For this review, take the finished solid that the model builds, in its own axes (mm). A direction names the side the tool comes from. Coordinates: 2 decimals unless noted, no trailing zeros. Write each loop counter-clockwise with the first axis right and the second up, starting at its lowest first coordinate (ties: lowest second). Pieces come first, ordered by that corner, then holes.
```python
from build123d import *

# Parameters (mm, degrees)
F0_W     = 19.05
F0_H     = 19.05
F1_DEPTH = 5.08
F2_W     = 16.51
F2_H     = 16.51
F3_DEPTH = 20.32
F5_DEPTH = 25.4
F6_SIZE  = 2.54
F7_SIZE  = 1.27


with BuildPart() as f1:
    # F0 (on Top) → F1 (new body)
    with BuildSketch(Plane.XY):
        with Locations((9.525, 9.525)):
            Rectangle(F0_W, F0_H)
    extrude(amount=F1_DEPTH)

    # F2 (on face) → F3 (join)
    with BuildSketch(Plane.XY.offset(5.08)):
        with Locations((9.525, 9.525)):
            Rectangle(F2_W, F2_H)
    extrude(amount=F3_DEPTH)

    # F4 (on face) → F5 (cut)
    with BuildSketch(Plane.XY.offset(25.4)):
        with BuildLine():
            Line((5.0348719395, 5.0348719395), (9.525, 9.525))
            Line((9.525, 9.525), (5.0348719395, 14.0151280605))
            ThreePointArc((5.0348719395, 14.0151280605), (3.175, 9.525), (5.0348719395, 5.0348719395))
        make_face()
        with BuildLine():
            Line((5.0348719395, 14.0151280605), (9.525, 9.525))
            Line((9.525, 9.525), (14.0151280605, 14.0151280605))
            ThreePointArc((14.0151280605, 14.0151280605), (9.525, 15.875), (5.0348719395, 14.0151280605))
        make_face()
        with BuildLine():
            Line((9.525, 9.525), (14.0151280605, 5.0348719395))
            ThreePointArc((14.0151280605, 5.0348719395), (15.3916350314, 7.0949602045), (15.875, 9.525))
            ThreePointArc((15.875, 9.525), (15.3916350314, 11.9550397955), (14.0151280605, 14.0151280605))
            Line((14.0151280605, 14.0151280605), (9.525, 9.525))
        make_face()
        with BuildLine():
            ThreePointArc((5.0348719395, 5.0348719395), (9.525, 3.175), (14.0151280605, 5.0348719395))
            Line((14.0151280605, 5.0348719395), (9.525, 9.525))
            Line((9.525, 9.525), (5.0348719395, 5.0348719395))
        make_face()
    extrude(amount=-F5_DEPTH, mode=Mode.SUBTRACT)

    # F6
    f6_edges = [f1.edges().sort_by_distance(p)[0] for p in [
        (17.78, 17.78, 15.24),
        (1.27, 17.78, 15.24),
        (1.27, 1.27, 15.24),
        (17.78, 1.27, 15.24),
    ]]
    chamfer(f6_edges, length=F6_SIZE)

    # F7
    f7_edges = [f1.edges().sort_by_distance(p)[0] for p in [
        (0, 0, 2.54),
        (0, 19.05, 2.54),
        (19.05, 19.05, 2.54),
        (19.05, 0, 2.54),
    ]]
    chamfer(f7_edges, length=F7_SIZE)


solid = f1.part
```
Q1. Add section C-C (z = 3.25). State the section outline as (x, y) points (3 decimals).
Ans:
outline: (0, 1.27) - (1.27, 0) - (17.78, 0) - (19.05, 1.27) - (19.05, 17.78) - (17.78, 19.05) - (1.27, 19.05) - (0, 17.78) - close; hole circle Ø12.7 at (9.525, 9.525)
Q2. For probe 1 along Y at (x, z) = (9.75, 3.5); probe 2 along X at (y, z) = (12, 19.25); probe 3 along X at (y, z) = (5, 1.75), list the stretches that pass through material, from the lowest coordinate up.
Ans:
probe 1: y = 0 to 3.18, 15.87 to 19.05
probe 2: x = 1.27 to 3.68, 15.37 to 17.78
probe 3: x = 0 to 5.07, 13.98 to 19.05
Q3. Add section B-B (x = 11.75). State the section outline as (y, z) points, then the cut area to 3 significant figures.
Ans:
outline: (0, 0) - (3.58, 0) - (3.58, 25.4) - (1.27, 25.4) - (1.27, 5.08) - (0, 5.08) - close; (15.47, 0) - (19.05, 0) - (19.05, 5.08) - (17.78, 5.08) - (17.78, 25.4) - (15.47, 25.4) - close
area: 130 mm2
Q4. Tool access review of faces 1 (the flat face through (1.27, 9, 15)), 2 (the flat face through (18, 10, 5.08)), 3 (the flat face through (16.53, 2.56, 15.1)): name each direction out of +Z, -Z, +X, -X, +Y, -Y from which nothing blocks a thin tool from reaching the whole face with its end or side.
Ans:
face 1: +Z, -X, +Y, -Y
face 2: +Z
face 3: +Z, +X, -Y
Q5. Clearance check with flat-ended pins moving along their axes: pin 1 Ø9 at (y, z) = (8.5, 11) entering from +X; pin 2 Ø9 at (x, z) = (7, 19.5) entering from -Y; pin 3 Ø1.5 at (y, z) = (12, 10.5) entering from -X. State where each tip first meets the part, or that it passes through.
Ans:
pin 1: stops at x = 17.78
pin 2: stops at y = 1.27
pin 3: stops at x = 1.27
Q6. Add section D-D (y = 16.5). State the section outline as (x, z) points.
Ans:
outline: (0, 0) - (19.05, 0) - (19.05, 5.08) - (16.52, 5.08) - (16.52, 25.4) - (2.53, 25.4) - (2.53, 5.08) - (0, 5.08) - close
Q7. Add section A-A (y = 12). State the section outline as (x, z) points.
Ans:
outline: (0, 0) - (3.68, 0) - (3.68, 25.4) - (1.27, 25.4) - (1.27, 5.08) - (0, 5.08) - close; (15.37, 0) - (19.05, 0) - (19.05, 5.08) - (17.78, 5.08) - (17.78, 25.4) - (15.37, 25.4) - close
